Autodesk Inventor part; units mm, degrees
ref_plane "YZ Plane" through (0, 0, 0) normal (1, 0, 0) x (0, 1, 0)
ref_plane "XZ Plane" through (0, 0, 0) normal (0, 1, 0) x (-1, 0, 0)
ref_plane "XY Plane" through (0, 0, 0) normal (0, 0, 1) x (1, 0, 0)
sketch "スケッチ1" plane through (0, 0, 0) normal (0, 0, 1) x (1, 0, 0)
  line L0 (0, 0) -> (0, 3.5)
  line L1 (0, 3.5) -> (0, 3.5)
  line L2 (0, 3.5) -> (0, 8)
  line L3 (0, 8) -> (8.3, 8)
  line L4 (8.3, 8) -> (8.3, 3)
  line L5 (8.3, 3) -> (5.8, 3)
  line L6 (5.8, 3) -> (5.8, 0)
  line L7 (5.8, 0) -> (0, 0)
  dimension "d0" = 3.5
  dimension "d1" = 3
  dimension "d2" = 2.5
  dimension "d4" = 0
  dimension "d5" = 8
  dimension "d34" = 5.8
revolve "回転1" add sketch "スケッチ1" angle 360 about axis through (5.8, 0, 0) along (-1, 0, 0)
sketch "スケッチ2" plane through (8.3, 0, 0) normal (1, 0, 0) x (0, 0, -1)
  point P0 (0, 0)
  point P1 (-5.5, 0)
  point P2 (5.5, 0)
  dimension "d10" = 5.5
  dimension "d11" = 5.5
hole "穴1" at (8.3, 0, 5.5) at (8.3, 0, -5.5) direction (-1, 0, 0) diameter 2.9 end through all counterbore diameter 5.5 counterbore depth 2.5
chamfer "面取り5" distance 0.5 angle 45 2 edges at (8.3, 3, 0) (8.3, -3, 0)
fillet "フィレット2" radius 0.5 8 edges at (6.8, 0.8377, -2.8807) (6.8, 0.8377, 2.8807) (6.8, -0.8377, 2.8807) (6.8, -0.8377, -2.8807) (7.05, 1.3765, -7.8807) (7.05, 1.3765, 7.8807) (7.05, -1.3765, 7.8807) (7.05, -1.3765, -7.8807)
properties part number "scara-base21" material "ABS プラスチック"
Build history of the part. All positions in model axes, mm. A direction names the side the tool comes from. Round coordinates to 2 decimals unless told otherwise and drop trailing zeros. Write each loop counter-clockwise with the first axis right and the second up, starting at its lowest first coordinate (ties: lowest second). Pieces come first, ordered by that corner, then holes. Notation, with made-up numbers: M -19.75,19.5 L 11.25,19.5 A17 ccw 11.25,45.5 Z; hole C -2.75,37 d6. An arc over 180 degrees is marked long. Use CSV: the item, a comma, the result in double quotes.
1. Flat gauge pins, fed straight in: pin 1 (1 mm diameter, centred on y = 5, z = 3, fed in from -X); pin 2 (1.5 mm diameter, centred on y = 2, z = -0.5, fed in from +X); pin 3 (1.5 mm diameter, centred on x = 5, y = 6, fed in from -Z); pin 4 (2 mm diameter, centred on x = 5.5, z = 3.5, fed in from -Y). Where does each tip first touch, or does it go through?
Reply:
pin 1,"stops at x = 0"
pin 2,"stops at x = 5.8"
pin 3,"stops at z = -6.04"
pin 4,"stops at y = -7.6"
2. Saw through at B-B (y = 0). Give the cut face in (x, z).
Reply:
outline,"M 0,-8 L 5.8,-8 L 5.8,-6.95 L 0,-6.95 Z; M 0,-4.05 L 5.8,-4.05 L 5.8,4.05 L 0,4.05 Z; M 0,6.95 L 5.8,6.95 L 5.8,8 L 0,8 Z"
3. Wall check: probe 1 along Z at (x, y) = (1.55, 0); probe 2 along Z at (x, y) = (3.25, 1); probe 3 along Y at (x, z) = (1.6, -5.5). Give the ranges that are in metal, low to high. Write a range as from..to.
Reply:
probe 1,"z = -8..-6.95, -4.05..4.05, 6.95..8"
probe 2,"z = -7.94..-6.55, -4.45..4.45, 6.55..7.94"
probe 3,"y = -5.81..-1.45, 1.45..5.81"
4. Tool access for faces 1 (the face through (7.94, 3.14, -0.05)), 2 (the face through (0, 0, 0)): list every direction of +Z, -Z, +X, -X, +Y, -Y with a clear straight run to the whole face (end or side of a thin tool).
Reply:
face 1,"+X"
face 2,"+Z, -Z, -X, +Y, -Y"
5. Saw through at C-C (x = 4). Give the cut face in (y, z), plus the area to 3 significant figures.
Reply:
outline,"C 0,0 d16; hole C 0,-5.5 d2.9; hole C 0,5.5 d2.9"
area,"188 mm²"
6. Two-plate mould, pull along Y, no slides. Class faces 3 (the face through (4.21, 7.39, -3.06)), 4 (the face through (7.033, -2.678, -4.873)), 5 (the face through (7, 3, 0)), 6 (the face through (8.3, -5, 0)): +Y half, -Y half, draft (parallel to the pull), parting line (faces both ways), or undercut.
Reply:
face 3,"parting line"
face 4,"undercut"
face 5,"undercut"
face 6,"draft"
7. Saw through at D-D (z = 0). Give the cut face in (x, y), plus the area to 3 significant figures.
Reply:
outline,"M 0,-8 L 8.3,-8 L 8.3,-3.5 L 7.8,-3 L 5.8,-3 L 5.8,3 L 7.8,3 L 8.3,3.5 L 8.3,8 L 0,8 Z"
area,"118 mm²"
